Autodesk Inventor part; units mm, degrees
ref_plane "YZ Plane" through (0, 0, 0) normal (1, 0, 0) x (0, 1, 0)
ref_plane "XZ Plane" through (0, 0, 0) normal (0, 1, 0) x (-1, 0, 0)
ref_plane "XY Plane" through (0, 0, 0) normal (0, 0, 1) x (1, 0, 0)
sketch "Sketch1" plane through (0, 0, 0) normal (0, 1, 0) x (-1, 0, 0)
  line L0 (0, 0) -> (30, 0)
  line L1 (30, 0) -> (30, -80)
  line L2 (30, -80) -> (0, -80)
  line L3 (0, -80) -> (0, 0)
  dimension "d0" = 30
  dimension "d1" = 80
extrude "Extrusion1" add sketch "Sketch1" along normal blind 2
sketch "Sketch2" plane through (0, 0, 0) normal (0, 0, 1) x (1, 0, 0)
  point P0 (0, 0)
sketch "Sketch3" plane through (0, 0, 0) normal (1, 0, 0) x (0, 1, 0)
  line L0 (0, 0) -> (50, 0)
  line L1 (50, 0) -> (50, -80)
  line L2 (50, -80) -> (0, -80)
  line L3 (0, -80) -> (0, 0)
  dimension "d4" = 50
  dimension "d11" = 80
extrude "Extrusion2" add sketch "Sketch3" along normal blind 2
sketch "Sketch4" plane through (0, 0, 0) normal (0, 1, 0) x (-1, 0, 0)
  point P0 (0, 0)
sketch "Sketch5" plane through (0, 0, 0) normal (-1, 0, 0) x (0, 0, 1)
  point P0 (0, 0)
sketch "Sketch6" plane through (0, 50, 0) normal (0, 1, 0) x (1, 0, 0)
  line L0 (-30, 0) -> (0, 0)
  line L1 (0, 0) -> (25, 0)
  line L2 (25, 0) -> (25, 80)
  line L3 (25, 80) -> (0, 80)
  line L4 (0, 80) -> (0, 0)
  dimension "d7" = 25
  dimension "d8" = 80
extrude "Extrusion3" add sketch "Sketch6" along normal blind 2
sketch "Sketch7" plane through (0, 2, 0) normal (0, 1, 0) x (1, 0, 0)
  point P0 (0, 0)
  point P1 (-20.3201, 56.529)
  point P2 (-18.421, 5.5073)
sketch "Sketch8" plane through (0, 0, 0) normal (0, -1, 0) x (1, 0, 0)
  point P0 (0, 0)
sketch "Sketch9" plane through (0, 50, 0) normal (0, -1, 0) x (1, 0, 0)
  line L0 (2, -80) -> (2, 0)
  line L1 (2, 0) -> (25, 0)
  line L2 (25, -80) -> (2, -80)
  point P0 (0, 0)
  point P1 (2, -65)
  point P2 (2, 0)
  point P3 (17.7309, -70)
  point P4 (17.7309, 0)
  point P5 (17.7309, -70)
  point P6 (17.7309, -5)
  dimension "d12" = 10
hole "Hole1" at (17.7309, 50, -70) at (17.7309, 50, -5) direction (0, 1, 0) diameter 2 depth 25 tip angle 118
sketch "Sketch10" plane through (2, 0, 0) normal (1, 0, 0) x (0, 0, -1)
  circle A0 centre (40, 26.2693) radius 10
  line L0 (80, 0) -> (80, 50)
  point P0 (0, 0)
  dimension "d20" = 20
  dimension "d21" = 40
extrude "Extrusion4" cut sketch "Sketch10" against normal blind 2
Check sheet for the modelled part. Datum: model origin and axes. Units: mm. A direction names the side the tool comes from. Give positions to 0.01 mm unless a question says otherwise; leave off trailing zeros. Write each loop counter-clockwise with the first axis right and the second up, starting at its lowest first coordinate (ties: lowest second). Pieces come first, ordered by that corner, then holes. Notation, with made-up numbers: (30, 3.25) -> (47, 3.25) arc R13 cw to (47, 19.25) -> close; hole circle Ø4 at (84, -36). An arc over 180 degrees is marked (long way). One line per item, written item: value. Start each with the question number.
Item 1: Section check C-C on z = -40. Record the cut outline in (x, y), then the cut area to 3 significant figures.
Item 2: Tool access check on faces 4 (the flat face through (-30, 1, -39)), 5 (the flat face through (13, 50, -41)). Record the directions out of +Z, -Z, +X, -X, +Y, -Y that give a thin tool (end or side, any length) a straight path to the whole face; none if there is none.
Item 3: Gauge pin test, flat ends, axial feed: pin 1 (1.6 mm diameter, centred on x = 17.73, z = -70, fed in from -Y); pin 2 (1.5 mm diameter, centred on x = -8, z = -63, fed in from +Y); pin 3 (25 mm diameter, centred on y = 26, z = -40, fed in from -X); pin 4 (25 mm diameter, centred on y = 37, z = -37.5, fed in from +X). Record the tip position at first contact, or that the pin passes through.
Item 4: Section check B-B on y = 34. Record the cut outline in (x, z), then the cut area to 3 significant figures.
Item 5: Section check D-D on x = 21. Record the cut outline in (y, z).
Item 6: Material ranges on probe 1 along X at (y, z) = (50.85, -70); probe 2 along X at (y, z) = (40.5, -17); probe 3 along Y at (x, z) = (13.5, -25), recorded low to high. Write a range as from..to.
Item 7: Section check A-A on z = -70. Record the cut outline in (x, y).
Item 8: Draft check along X on faces 1 (the cylindrical face through (17.7, 51, -69)), 2 (the flat face through (0, 32, -49)), 3 (the flat face through (-15, 2, -39)). Enter one of: +X half, -X half, draft (parallel to the pull), parting line (faces both ways), or undercut.
Results list:
1. outline: (-30, 0) -> (2, 0) -> (2, 16.27) -> (0, 16.27) -> (0, 2) -> (-30, 2) -> close; (0, 36.27) -> (2, 36.27) -> (2, 50) -> (25, 50) -> (25, 52) -> (0, 52) -> close
1. area: 170 mm²
2. face 4: +Z, -Z, -X, +Y, -Y
2. face 5: +Z, -Z, +X, -Y
3. pin 1: through
3. pin 2: y = 2
3. pin 3: x = 0
3. pin 4: x = 2
4. outline: (0, -80) -> (2, -80) -> (2, -46.34) -> (0, -46.34) -> close; (0, -33.66) -> (2, -33.66) -> (2, 0) -> (0, 0) -> close
4. area: 135 mm²
5. outline: (50, -80) -> (52, -80) -> (52, 0) -> (50, 0) -> close
6. probe 1: 0..16.73, 18.73..25
6. probe 2: 0..2
6. probe 3: 50..52
7. outline: (-30, 0) -> (2, 0) -> (2, 50) -> (16.73, 50) -> (16.73, 52) -> (0, 52) -> (0, 2) -> (-30, 2) -> close; (18.73, 50) -> (25, 50) -> (25, 52) -> (18.73, 52) -> close
8. face 1: undercut
8. face 2: -X half
8. face 3: draft
